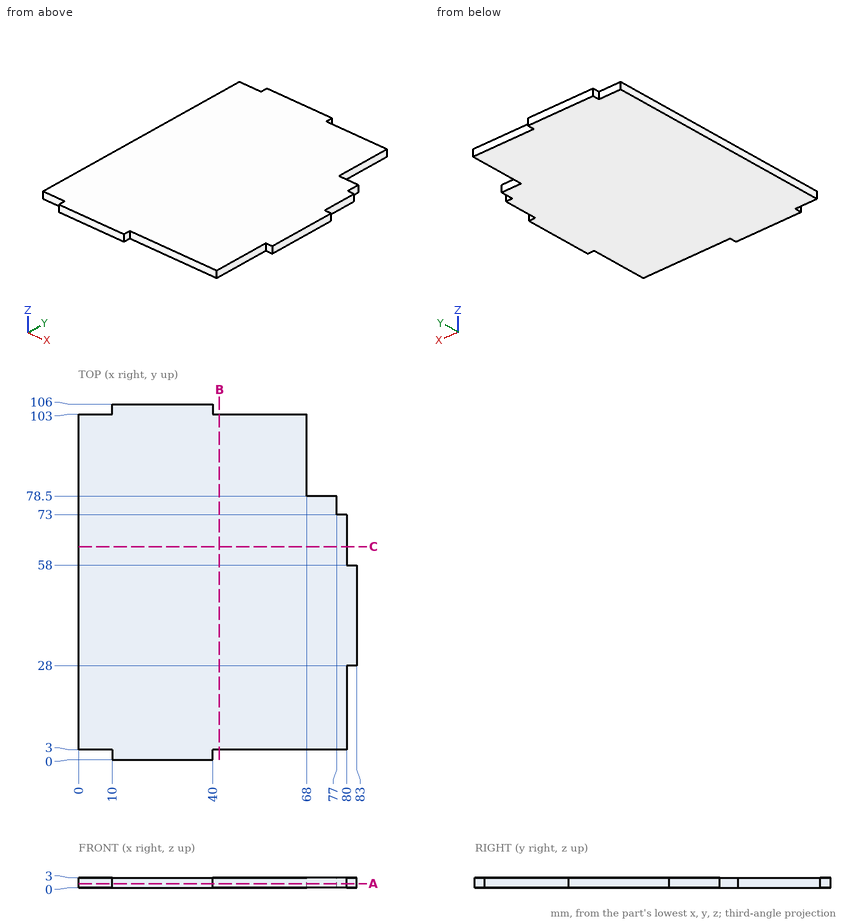
Could you check a few things on this drawing? It's one solid part, dimensions in mm from its lowest x, y, z. Coordinates: 2 decimals unless noted, no trailing zeros. Order: outer loops, then holes, each group sorted by start corner. A loop starts at its lowest first (then second) coordinate and runs counter-clockwise, first axis right, second up. Notation, with made-up numbers: M 79,89 L 100,89 A11 cw 100,106 Z; hole C -0.75,39 d2. An arc over 180 degrees is marked long. Use one line per item in the form item = value. Start each with the question number.
1. Suppose I cut it at A-A on z = 1.2. Write out the boundary of the cut face in (x, y), then the cut area to 3 significant figures.
2. For pin 1 (1.5 mm diameter, centred on x = 45.5, y = 79.5, fed in from -Z); pin 2 (1.5 mm diameter, centred on x = 70.5, z = 2, fed in from +Y); pin 3 (0.9 mm diameter, centred on y = 105, z = 1.5, fed in from +X); pin 4 (0.9 mm diameter, centred on x = 78, z = 2, fed in from +Y), each with a flat end and sliding along its axis, tell me the tip position at first contact or that it passes through.
3. Please list where these lines run through material, in increasing order: line 1 (X direction, y = 26, z = 0.9); line 2 (Y direction, x = 60, z = 2.7); line 3 (Y direction, x = 74, z = 2.85).
4. Suppose I cut it at B-B on x = 42. Write out the boundary of the cut face in (y, z).
5. Suppose I cut it at C-C on y = 63.5. Write out the boundary of the cut face in (x, z).
Geometry says:
q1.outline = M 0,3 L 10,3 L 10,0 L 40,0 L 40,3 L 80,3 L 80,28 L 83,28 L 83,58 L 80,58 L 80,73 L 77,73 L 77,78.5 L 68,78.5 L 68,103 L 40,103 L 40,106 L 10,106 L 10,103 L 0,103 Z
q1.area = 7,960 mm^2
q2.pin_1 = 0
q2.pin_2 = 78.5
q2.pin_3 = 40
q2.pin_4 = 73
q3.line_1 = 0 to 80
q3.line_2 = 3 to 103
q3.line_3 = 3 to 78.5
q4.outline = M 3,0 L 103,0 L 103,3 L 3,3 Z
q5.outline = M 0,0 L 80,0 L 80,3 L 0,3 Z
